The listing builds one solid part. Answer for the finished solid, in the listing's coordinates (mm). Round coordinates to 2 decimals unless told otherwise and drop trailing zeros. Order: outer loops, then holes, each group sorted by start corner. A loop starts at its lowest first (then second) coordinate and runs counter-clockwise, first axis right, second up. Notation, with made-up numbers: (38.5, 7) - (96.5, 7) arc R20 cw to (96.5, 43) - close; hole circle Ø10 at (1.5, 9.5). An arc over 180 degrees is marked (long way). One line per item, written item: value. Start each with the question number.
1. Flat-ended cylindrical pins translate along their axes: P1, Ø2, axis at x = 29.2, z = 15, coming from the -Y side; P2, Ø4, axis at x = -29.2, z = -15, coming from the +Y side. Find the tip coordinate at first contact, or state that the pin passes through.
2. Section C-C, the plane z = -15 is taken. Give the vertices of the cut face in (x, y), then the cut area to 3 significant figures.
3. Straight lines are drawn through the part: line 1 (Z direction, x = -29.2, y = -0.5); line 2 (X direction, y = -0.4, z = 15); line 3 (Z direction, x = -29, y = 1.65). For each, find the intervals that lie inside material, in ascending order.
4. Section A-A, the plane y = -0.45 is taken. Give the vertices of the cut face in (x, z), then the cut area to 3 significant figures.
5. Section B-B, the plane x = -29.2 is taken. Give the vertices of the cut face in (y, z), then the cut area to 3 significant figures.
from build123d import *

# Parameters (mm, degrees)
SKETCH1_W                                           = 66
SKETCH1_H                                           = 37.5
BOSS_EXTRUDE1_DEPTH                                 = 2
CSK_FOR_M3_COUNTERSUNK_FLAT_HEAD_SCREW1_D           = 3.6
CSK_FOR_M3_COUNTERSUNK_FLAT_HEAD_SCREW1_DEPTH       = 5
CSK_FOR_M3_COUNTERSUNK_FLAT_HEAD_SCREW1_CSINK_D     = 6.3
CSK_FOR_M3_COUNTERSUNK_FLAT_HEAD_SCREW1_CSINK_ANGLE = 90
CSK_FOR_M3_COUNTERSUNK_FLAT_HEAD_SCREW1_TIP         = 1.081549114


with BuildPart() as part:
    # Sketch1 → Boss-Extrude1 (new, symmetric)
    with BuildSketch(Plane(origin=(0, 0, 0), x_dir=(1, 0, 0), z_dir=(0, 1, 0))):
        Rectangle(SKETCH1_W, SKETCH1_H)
    extrude(amount=BOSS_EXTRUDE1_DEPTH, both=True)

    # CSK for M3 Countersunk Flat Head Screw1
    with Locations(Plane(origin=(0, 2, 0), x_dir=(1, 0, 0), z_dir=(0, 1, 0))):
        with Locations((-29.2, -15), (-29.2, 15), (29.2, 15), (29.2, -15)):
            CounterSinkHole(CSK_FOR_M3_COUNTERSUNK_FLAT_HEAD_SCREW1_D / 2, CSK_FOR_M3_COUNTERSUNK_FLAT_HEAD_SCREW1_CSINK_D / 2, depth=CSK_FOR_M3_COUNTERSUNK_FLAT_HEAD_SCREW1_DEPTH, counter_sink_angle=CSK_FOR_M3_COUNTERSUNK_FLAT_HEAD_SCREW1_CSINK_ANGLE)
            with Locations((0, 0, -(CSK_FOR_M3_COUNTERSUNK_FLAT_HEAD_SCREW1_DEPTH + CSK_FOR_M3_COUNTERSUNK_FLAT_HEAD_SCREW1_TIP / 2))):  # 118° drill point
                Cone(0, CSK_FOR_M3_COUNTERSUNK_FLAT_HEAD_SCREW1_D / 2, CSK_FOR_M3_COUNTERSUNK_FLAT_HEAD_SCREW1_TIP, mode=Mode.SUBTRACT)


solid = part.part
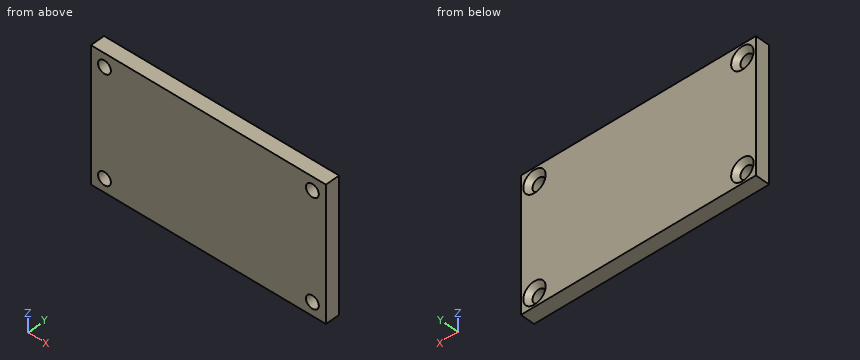
Answer list:
1. P1: passes through
1. P2: stops at y = 0.85
2. outline: (-33, -2) - (-31, -2) - (-31, 0.65) - (-32.35, 2) - (-33, 2) - close; (-27.4, -2) - (27.4, -2) - (27.4, 0.65) - (26.05, 2) - (-26.05, 2) - (-27.4, 0.65) - close; (31, -2) - (33, -2) - (33, 2) - (32.35, 2) - (31, 0.65) - close
2. area: 232 mm²
3. line 1: z = -18.75 to -16.8, -13.2 to 13.2, 16.8 to 18.75
3. line 2: x = -33 to -31, -27.4 to 27.4, 31 to 33
3. line 3: z = -18.75 to -17.79, -12.21 to 12.21, 17.79 to 18.75
4. outline: (-33, -18.75) - (33, -18.75) - (33, 18.75) - (-33, 18.75) - close; hole circle Ø3.6 at (-29.2, -15); hole circle Ø3.6 at (-29.2, 15); hole circle Ø3.6 at (29.2, -15); hole circle Ø3.6 at (29.2, 15)
4. area: 2,430 mm²
5. outline: (-2, -18.75) - (2, -18.75) - (2, -18.15) - (0.65, -16.8) - (-2, -16.8) - close; (-2, -13.2) - (0.65, -13.2) - (2, -11.85) - (2, 11.85) - (0.65, 13.2) - (-2, 13.2) - close; (-2, 16.8) - (0.65, 16.8) - (2, 18.15) - (2, 18.75) - (-2, 18.75) - close
5. area: 118 mm²
